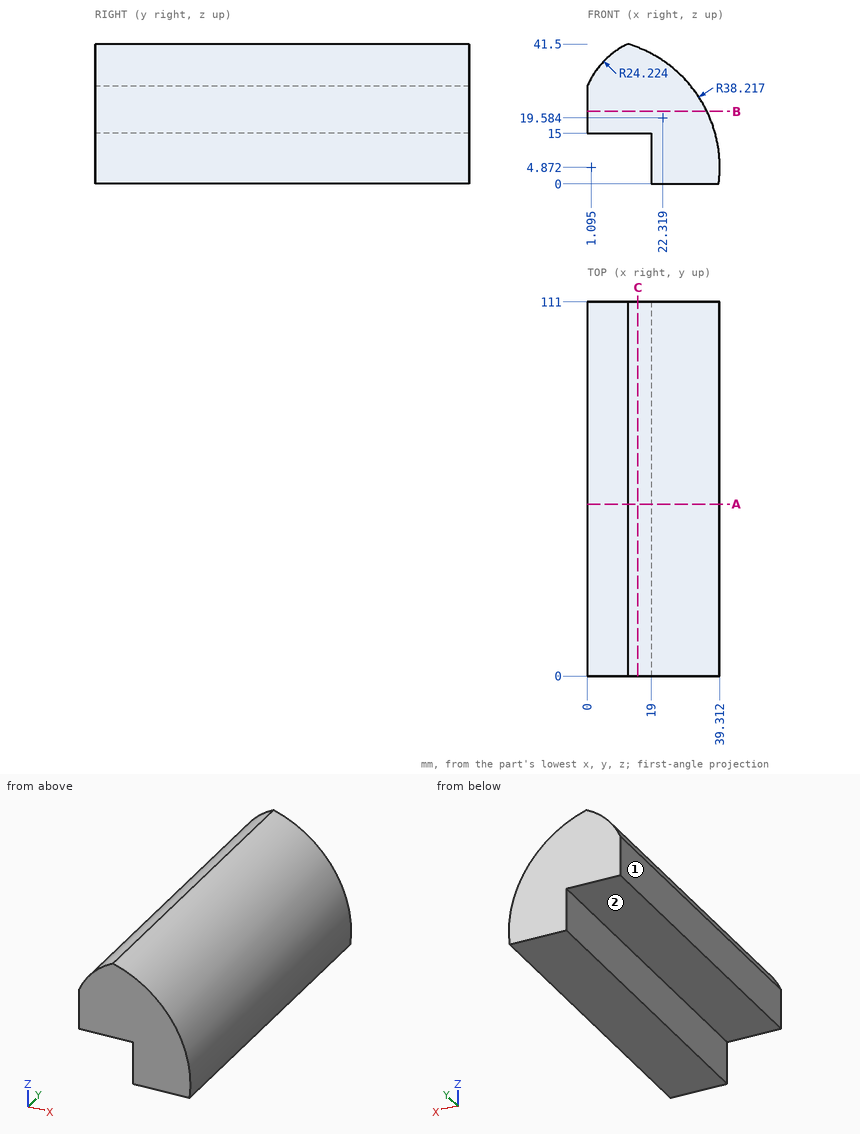
The figure shows three views and two pictorial views of one solid part (mm, origin at its lowest corner). Answer the questions. A direction names the side the tool comes from. Coordinates: 2 decimals unless noted, no trailing zeros. Order: outer loops, then holes, each group sorted by start corner. A loop starts at its lowest first (then second) coordinate and runs counter-clockwise, first axis right, second up.
Q1. A cutting plane is placed at B-B, the plane z = 21.5. Write down the section's boundary in (x, y) (1 decimal), and give its area (3 significant figures).
Q2. Given P1, Ø15, axis at x = 10, y = 61, coming from the -Z side; P2, Ø8, axis at x = 35, y = 79, coming from the +Z side; P3, Ø7.5, axis at y = 70, z = 9, coming from the -X side, each flat-ended and moving along its own axis, determine where each tip first touches the part or whether it passes through.
Q3. Consider line 1 (X direction, y = 83, z = 3.5); line 2 (X direction, y = 54, z = 23); line 3 (Z direction, x = 9, y = 65). Determine where each line is inside the solid, lowest interval first.
Q4. A cutting plane is placed at C-C, the plane x = 15. Write down the section's boundary in (y, z), and give its area (3 significant figures).
Q5. A cutting plane is placed at A-A, the plane y = 51. Write down the section's boundary in (x, z) (1 decimal), and give its area (3 significant figures).
Q6. Which of the six approach directions +Z, -Z, +X, -X, +Y, -Y give full straight-line access (tool end or side, diameter ignored) to the marked faces 1 and 2?
Answers follow:
1. outline: (0, 0) - (35.5, 0) - (35.5, 111) - (0, 111) - close
1. area: 3,940 mm2
2. P1: stops at z = 15
2. P2: stops at z = 28.67
2. P3: stops at x = 19
3. line 1: x = 19 to 39.29
3. line 2: x = 0 to 34.74
3. line 3: z = 15 to 39.82
4. outline: (0, 15) - (111, 15) - (111, 40.47) - (0, 40.47) - close
4. area: 2,830 mm2
5. outline: (0, 15) - (19, 15) - (19, 0) - (39, 0) arc R38.2 ccw to (12, 41.5) arc R24.2 ccw to (0, 29) - close
5. area: 1,030 mm2
6. face 1: +Z, -Z, -X, +Y, -Y
6. face 2: -Z, -X, +Y, -Y
